Answer from the drawing. Dimensions are ordinates in mm from the lowest x, y and z of the part. A direction names the side the tool comes from. Coordinates: 2 decimals unless noted, no trailing zeros. Order: outer loops, then holes, each group sorted by start corner. A loop starts at its lowest first (then second) coordinate and runs counter-clockwise, first axis right, second up. Notation, with made-up numbers: (22.5, -37) - (61.5, -37) arc R10 ccw to (61.5, -29) - close; hole circle Ø6 at (84.25, 31.25). An arc over 180 degrees is marked (long way). One line per item, written item: value. Start each with the question number.
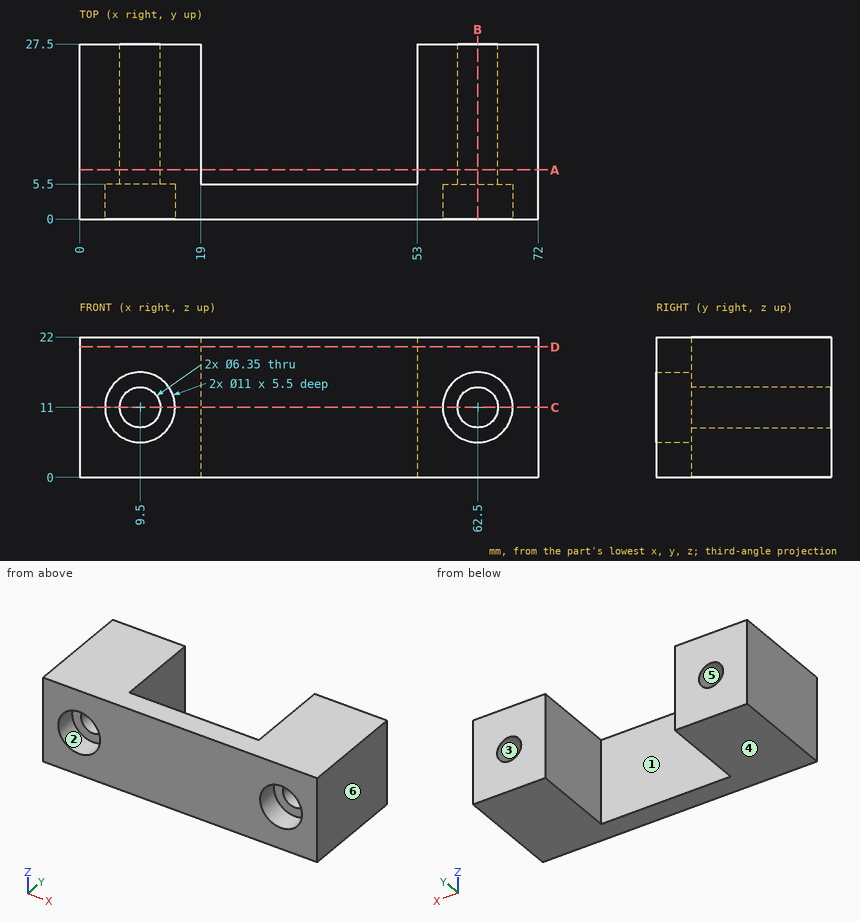
(1) The part is cut by section B-B on x = 62.5. Determine the outline of the cut face in (y, z) (3 decimals), plus the area to 3 significant figures.
(2) The part is cut by section A-A on y = 7.75. Determine the outline of the cut face in (x, z) (3 decimals), plus the area to 3 significant figures.
(3) For the marked faces 1, 2 and 3, determine the directions among +Z, -Z, +X, -X, +Y, -Y from which every point of the face is accessible in a straight line to the end or side of a thin tool.
(4) Flat-ended cylindrical pins translate along their axes: pin 1 Ø10 at (x, z) = (47.5, 7.5) entering from +Y; pin 2 Ø10 at (x, z) = (9.5, 11) entering from -Y. Find the tip coordinate at first contact, or state that the pin passes through.
(5) Consider probe 1 along X at (y, z) = (18, 11) (3 decimals); probe 2 along X at (y, z) = (3.85, 11); probe 3 along X at (y, z) = (7, 19.25). Determine where each line is inside the solid, lowest interval first.
(6) The part is cut by section C-C on z = 11. Determine the outline of the cut face in (x, y) (3 decimals), plus the area to 3 significant figures.
(7) For a pull along Z with two mould halves and no side action, classify the marked faces 4, 5 and 6 as pulls with the +Z half, pulls with the -Z half, needs draft (parallel to the pull), parting line crosses it, or undercut.
(8) The part is cut by section D-D on z = 20.5. Determine the outline of the cut face in (x, y).
Completed:
1. outline: (0, 0) - (27.5, 0) - (27.5, 7.825) - (5.5, 7.825) - (5.5, 5.5) - (0, 5.5) - close; (0, 16.5) - (5.5, 16.5) - (5.5, 14.175) - (27.5, 14.175) - (27.5, 22) - (0, 22) - close
1. area: 405 mm2
2. outline: (0, 0) - (19, 0) - (19, 22) - (0, 22) - close; (53, 0) - (72, 0) - (72, 22) - (53, 22) - close; hole circle Ø6.35 at (9.5, 11); hole circle Ø6.35 at (62.5, 11)
2. area: 773 mm2
3. face 1: +Z, -Z, +Y
3. face 2: -Y
3. face 3: +Y, -Y
4. pin 1: stops at y = 5.5
4. pin 2: stops at y = 5.5
5. probe 1: x = 0 to 6.325, 12.675 to 19, 53 to 59.325, 65.675 to 72
5. probe 2: x = 0 to 4, 15 to 57, 68 to 72
5. probe 3: x = 0 to 19, 53 to 72
6. outline: (0, 0) - (4, 0) - (4, 5.5) - (6.325, 5.5) - (6.325, 27.5) - (0, 27.5) - close; (12.675, 5.5) - (15, 5.5) - (15, 0) - (57, 0) - (57, 5.5) - (59.325, 5.5) - (59.325, 27.5) - (53, 27.5) - (53, 5.5) - (19, 5.5) - (19, 27.5) - (12.675, 27.5) - close; (65.675, 5.5) - (68, 5.5) - (68, 0) - (72, 0) - (72, 27.5) - (65.675, 27.5) - close
6. area: 832 mm2
7. face 4: pulls with the -Z half
7. face 5: undercut
7. face 6: needs draft
8. outline: (0, 0) - (72, 0) - (72, 27.5) - (53, 27.5) - (53, 5.5) - (19, 5.5) - (19, 27.5) - (0, 27.5) - close
